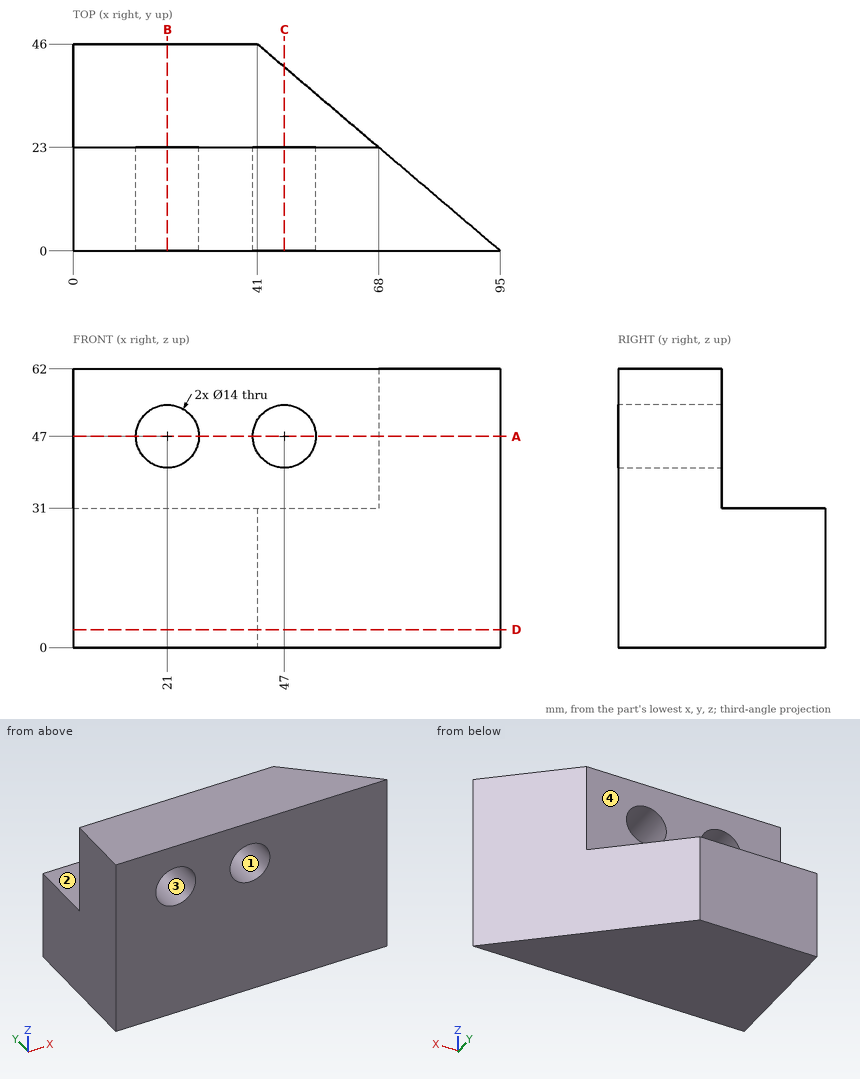
Geometry: see drawing. Coordinates: mm, zero at the bounding-box minimum. Coordinates: 2 decimals unless noted, no trailing zeros. Loops run counter-clockwise (first coordinate to the right, second up) from the corner with the lowest first, then second, coordinate; pieces in that order, holes last. Notation, with made-up numbers: M 4.25,18.5 L 37.25,18.5 A12 cw 37.25,32.5 Z; hole C 86.5,39.25 d8. An arc over 180 degrees is marked long. Answer in a Markdown table with one row per item.
1. Section C-C, the plane x = 47. Output: boundary loops of the cut face in (y, z).
Response:
| item | result |
|---|---|
| outline | M 0,0 L 40.89,0 L 40.89,31 L 23,31 L 23,40 L 0,40 Z; M 0,54 L 23,54 L 23,62 L 0,62 Z |
2. Section A-A, the plane z = 47. Output: boundary loops of the cut face in (x, y).
Response:
| item | result |
|---|---|
| outline | M 0,0 L 14,0 L 14,23 L 0,23 Z; M 28,0 L 40,0 L 40,23 L 28,23 Z; M 54,0 L 95,0 L 68,23 L 54,23 Z |
3. Material intervals for line 1 (X direction, y = 18, z = 47); line 2 (X direction, y = 20.5, z = 51); line 3 (Z direction, x = 18.5, y = 32.5), sorted ascending.
Response:
| item | result |
|---|---|
| line 1 | x = 0 to 14, 28 to 40, 54 to 73.87 |
| line 2 | x = 0 to 15.26, 26.74 to 41.26, 52.74 to 70.93 |
| line 3 | z = 0 to 31 |
4. First-contact query: pin 1 (18 mm diameter, centred on x = 21, z = 47, fed in from +Y); pin 2 (3 mm diameter, centred on x = 30, y = 31, fed in from +Z); pin 3 (8.5 mm diameter, centred on x = 47, z = 47, fed in from -Y); pin 4 (3 mm diameter, centred on y = 11.5, z = 55, fed in from +X). Flat tips, straight axial feed; report the tip coordinate or a pass-through.
Response:
| item | result |
|---|---|
| pin 1 | stops at y = 23 |
| pin 2 | stops at z = 31 |
| pin 3 | passes through |
| pin 4 | stops at x = 83.26 |
5. Section D-D, the plane z = 4. Output: boundary loops of the cut face in (x, y).
Response:
| item | result |
|---|---|
| outline | M 0,0 L 95,0 L 41,46 L 0,46 Z |
6. Section B-B, the plane x = 21. Output: boundary loops of the cut face in (y, z), then the cut area to 3 significant figures.
Response:
| item | result |
|---|---|
| outline | M 0,0 L 46,0 L 46,31 L 23,31 L 23,40 L 0,40 Z; M 0,54 L 23,54 L 23,62 L 0,62 Z |
| area | 1,820 mm2 |
7. Draft query along Z for the marked faces 1, 2, 3 and 4. Return one class per face: pulls with the +Z half, pulls with the -Z half, needs draft (parallel to the pull), parting line crosses it, or undercut.
Response:
| item | result |
|---|---|
| face 1 | undercut |
| face 2 | pulls with the +Z half |
| face 3 | undercut |
| face 4 | needs draft |
